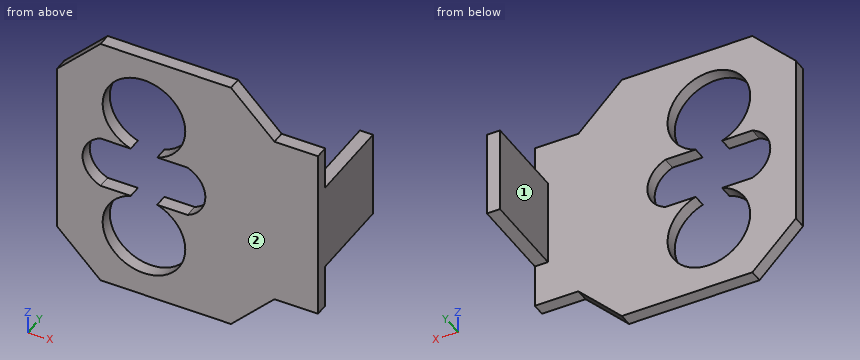
Autodesk Inventor part; units mm, degrees
ref_plane "YZ Plane" through (0, 0, 0) normal (1, 0, 0) x (0, 1, 0)
ref_plane "XZ Plane" through (0, 0, 0) normal (0, 1, 0) x (-1, 0, 0)
ref_plane "XY Plane" through (0, 0, 0) normal (0, 0, 1) x (1, 0, 0)
sketch "Sketch1" plane through (0, 0, 0) normal (0, 1, 0) x (-1, 0, 0)
  line L0 (0, 0) -> (30, 0)
  line L1 (0, 0) -> (-30, 0)
  line L2 (30, 0) -> (-10, 0)
  line L3 (-10, 0) -> (-10, 30)
  line L4 (-10, 0) -> (-10, -30)
  line L5 (-10, 30) -> (20, 30)
  line L6 (-10, -30) -> (20, -30)
  line L7 (20, 30) -> (20, -30)
  line L8 (30, 0) -> (30, 20)
  line L9 (30, 0) -> (30, -20)
  line L10 (30, 20) -> (20, 30)
  line L11 (30, -20) -> (20, -30)
  line L12 (-30, 0) -> (-30, 20)
  line L13 (-30, 0) -> (-30, -20)
  line L14 (-30, 20) -> (-20, 20)
  line L15 (-20, 20) -> (-10, 30)
  line L16 (-30, -20) -> (-20, -20)
  line L17 (-20, -20) -> (-10, -30)
  line L18 (20, 0) -> (20, 6)
  line L19 (20, 0) -> (20, -6)
  arc A0 (20, -6) -> (20, 6) centre (17.6853, 0) ccw
  line L20 (0, 0) -> (0, 6)
  line L21 (0, 0) -> (0, -6)
  arc A1 (0, 6) -> (0, -6) centre (2.3147, 0) ccw
  line L22 (0, 30) -> (10, 30)
  circle A2 centre (10.0225, 15.038) radius 9
  line L23 (0, -30) -> (10, -30)
  circle A3 centre (10, -15) radius 9
  line L24 (20, 6) -> (20, -6)
  line L25 (20, 6) -> (0, 6)
  line L26 (20, -6) -> (0, -6)
  point P0 (10, -6)
  dimension "d0" = 30
  dimension "d1" = 30
  dimension "d2" = 40
  dimension "d5" = 30
  dimension "d6" = 30
  dimension "d8" = 30
  dimension "d9" = 30
  dimension "d10" = 20
  dimension "d11" = 20
  dimension "d12" = 20
  dimension "d13" = 20
  dimension "d14" = 10
  dimension "d15" = 10
  dimension "d16" = 6
  dimension "d17" = 6
  dimension "d18" = 6.431
  dimension "d19" = 6
  dimension "d20" = 6
  dimension "d22" = 6.431
  dimension "d25" = 18
  dimension "d28" = 18
extrude "Extrusion1" add sketch "Sketch1" along normal blind 3 contours A1 L26 L7 L6 L4 L1 | L1 L3 L5 L7 L25 A1 | A0 L7 L10 L8 L0 | L0 L9 L11 L7 A0 | L4 L17 L16 L13 L1 | L1 L12 L14 L15 L3
sketch "Sketch2" plane through (0, 3, 0) normal (0, 1, 0) x (1, 0, 0)
  line L0 (30, 10) -> (30, -10)
  line L1 (30, 10) -> (27, 10)
  line L2 (27, 10) -> (27, -10)
  line L3 (27, -10) -> (30, -10)
  line L4 (-19, -30) -> (-10, -30)
  circle A0 centre (-10, -15) radius 9.5
  circle A1 centre (-10, 15) radius 9.5
  point P0 (0, 0)
  dimension "d34" = 20
  dimension "d35" = 3
  dimension "d37" = 19
  dimension "d39" = 19
hole "Hole1" at (-10, 3, 15) direction (0, -1, 0) diameter 19 end through all
hole "Hole2" at (-10, 3, -15) direction (0, -1, 0) diameter 19 end through all
sketch "Sketch3" plane through (0, 3, 0) normal (0, 1, 0) x (1, 0, 0)
  line L0 (30, 10) -> (30, -10)
  line L1 (30, -10) -> (27, -10)
  line L2 (27, -10) -> (27, 10)
  line L3 (27, 10) -> (30, 10)
  point P0 (0, 0)
extrude "Extrusion2" add sketch "Sketch3" along normal blind 20
properties part number "Ultrasonic_Body"
Verification items for the finished model (mm, model axes). Face numbers are marked on the shaded views. A direction names the side the tool comes from. Coordinates: 2 decimals unless noted, no trailing zeros. Order: outer loops, then holes, each group sorted by start corner. A loop starts at its lowest first (then second) coordinate and runs counter-clockwise, first axis right, second up.
1. Go/stop test with flat-tipped pins: pin 1 Ø2.5 at (x, y) = (29, 14) entering from -Z; pin 2 Ø6 at (y, z) = (8, -1.5) entering from -X; pin 3 Ø5 at (x, z) = (3, -5.5) entering from +Y; pin 4 Ø12 at (y, z) = (5, 10.5) entering from +X. Record where each tip stops, or that it passes through.
Results found:
pin 1: stops at z = -10
pin 2: stops at x = 27
pin 3: stops at y = 3
pin 4: stops at x = 30
2. Sectioned sample at B-B, the plane z = -15. Record the cut outline in (x, y).
Results found:
outline: (-30, 0) - (-19.5, 0) - (-19.5, 3) - (-30, 3) - close; (-0.5, 0) - (30, 0) - (30, 3) - (-0.5, 3) - close
3. Sectioned sample at C-C, the plane x = -3. Record the cut outline in (y, z), and give its area (3 significant figures).
Results found:
outline: (0, -30) - (3, -30) - (3, -21.42) - (0, -21.42) - close; (0, -8.58) - (3, -8.58) - (3, -6) - (0, -6) - close; (0, 6) - (3, 6) - (3, 8.58) - (0, 8.58) - close; (0, 21.42) - (3, 21.42) - (3, 30) - (0, 30) - close
area: 66.9 mm2
4. Scan lines: line 1 (Z direction, x = -10, y = 0.7); line 2 (X direction, y = 2.3, z = -15); line 3 (Y direction, x = -24, z = 23). Record each from-to range of solid material in increasing order.
Results found:
line 1: z = -30 to -24.5, 24.5 to 30
line 2: x = -30 to -19.5, -0.5 to 30
line 3: y = 0 to 3
5. Sectioned sample at A-A, the plane x = -10. Record the cut outline in (y, z).
Results found:
outline: (0, -30) - (3, -30) - (3, -24.5) - (0, -24.5) - close; (0, 24.5) - (3, 24.5) - (3, 30) - (0, 30) - close
6. Set-up check for the marked faces 1 and 2: record each of +Z, -Z, +X, -X, +Y, -Y from which the full face is reachable in a straight line by a thin tool's end or side.
Results found:
face 1: +Z, -Z, -X, +Y
face 2: +Z, -Z, +X, -X, -Y
7. Sectioned sample at D-D, the plane y = 13.5. Record the cut outline in (x, z), and give its area (3 significant figures).
Results found:
outline: (27, -10) - (30, -10) - (30, 10) - (27, 10) - close
area: 60.0 mm2
